Geometry: final body of the model. Coordinates: model frame, mm. Coordinates: 2 decimals unless noted, no trailing zeros. Write each loop counter-clockwise with the first axis right and the second up, starting at its lowest first coordinate (ties: lowest second). Pieces come first, ordered by that corner, then holes. Notation, with made-up numbers: (15.5, -35.75) -> (49.5, -35.75) arc R12 cw to (49.5, -28.75) -> close; hole circle Ø2 at (68.25, 79). An arc over 180 degrees is marked (long way). Answer as a JSON object with one key per item and string values. Group by question number.
```python
from build123d import *

# Parameters (mm, degrees)
SKETCH1_R               = 9
SKETCH1_R_2             = 3
BOSS_EXTRUDE1_DEPTH     = 132
SKETCH2_R               = 6
CUT_EXTRUDE1_DEPTH      = 10
CUT_EXTRUDE1_DEPTH_BACK = 10


with BuildPart() as part:
    # Sketch1 → Boss-Extrude1 (new body)
    with BuildSketch(Plane.XY):
        Circle(SKETCH1_R)
        Circle(SKETCH1_R_2, mode=Mode.SUBTRACT)
    extrude(amount=BOSS_EXTRUDE1_DEPTH)

    # Sketch2 → Cut-Extrude1 (cut, two sides)
    with BuildSketch(Plane(origin=(0, 0, 0), x_dir=(1, 0, 0), z_dir=(0, 1, 0))) as cut_extrude1_sk:
        with Locations((0, -66)):
            Circle(SKETCH2_R)
    extrude(amount=CUT_EXTRUDE1_DEPTH, mode=Mode.SUBTRACT)
    extrude(cut_extrude1_sk.sketch, amount=-CUT_EXTRUDE1_DEPTH_BACK, mode=Mode.SUBTRACT)


solid = part.part
```
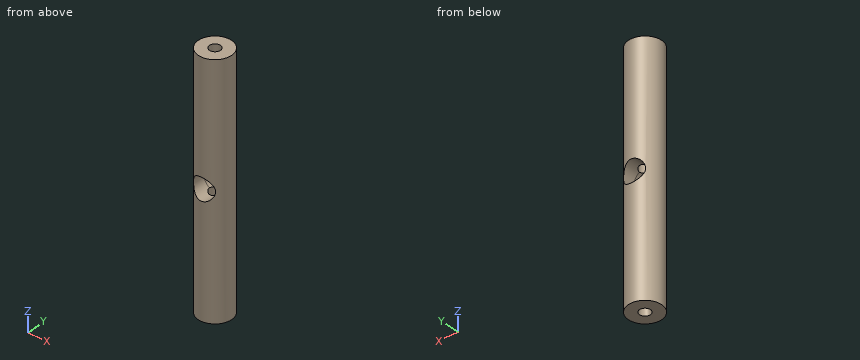
Item 1: Ray query, L1, parallel to Z at x = 0, y = -6; L2, parallel to Y at x = 0, z = 36.5; L3, parallel to X at y = -0.25, z = 6. Return the intervals inside material, ascending. Write a range as [from, to].
Item 2: Section B-B on y = -1.25. Output: boundary loops of the cut face in (x, z), then the cut area to 3 significant figures.
Item 3: Contact query for flat-ended pins moving along their axis: pin 1 (3 mm diameter, centred on y = -6, z = 62, fed in from -X); pin 2 (9.5 mm diameter, centred on x = 0, z = 66, fed in from +Y); pin 3 (3 mm diameter, centred on x = -4, z = 56.5, fed in from +Y); pin 4 (3 mm diameter, centred on y = -5, z = 106.5, fed in from +X). Output: stop coordinate, or through.
Item 4: Section D-D on z = 66. Output: boundary loops of the cut face in (x, y).
Item 5: Section C-C on z = 95. Output: boundary loops of the cut face in (x, y), then the cut area to 3 significant figures.
Item 6: Section A-A on x = 0. Output: boundary loops of the cut face in (y, z).
Answer sheet:
{
 "1": {"L1": "z = [0, 60], [72, 132]", "L2": "y = [-9, -3], [3, 9]", "L3": "x = [-9, -2.99], [2.99, 9]"},
 "2": {"outline": "(-8.91, 0) -> (-2.73, 0) -> (-2.73, 60.66) arc R6 cw to (-2.73, 71.34) -> (-2.73, 132) -> (-8.91, 132) -> close; (2.73, 0) -> (8.91, 0) -> (8.91, 132) -> (2.73, 132) -> (2.73, 71.34) arc R6 cw to (2.73, 60.66) -> close", "area": "1,580 mm^2"},
 "3": {"pin 1": "stops at x = -7.79", "pin 2": "passes through", "pin 3": "stops at y = 8.65", "pin 4": "stops at x = 8.29"},
 "4": {"outline": "(-6, -6.71) -> (-6, 6.71) arc R9 ccw to start; (6, -6.71) arc R9 ccw to (6, 6.71) -> close"},
 "5": {"outline": "circle Ø18 at (0, 0); hole circle Ø6 at (0, 0)", "area": "226 mm^2"},
 "6": {"outline": "(-9, 0) -> (-3, 0) -> (-3, 60) -> (-9, 60) -> close; (-9, 72) -> (-3, 72) -> (-3, 132) -> (-9, 132) -> close; (3, 0) -> (9, 0) -> (9, 60) -> (3, 60) -> close; (3, 72) -> (9, 72) -> (9, 132) -> (3, 132) -> close"}
}
